Build history of the part. All positions in model axes, mm. A direction names the side the tool comes from. Coordinates: 2 decimals unless noted, no trailing zeros. Loops run counter-clockwise (first coordinate to the right, second up) from the corner with the lowest first, then second, coordinate; pieces in that order, holes last. Notation, with made-up numbers: (-23.75, 56) - (27.25, 56) arc R30 cw to (27.25, 90) - close; hole circle Ø1 at (-5, 38.5). An arc over 180 degrees is marked (long way). One line per item, written item: value.
Autodesk Inventor part; units mm, degrees
ref_plane "YZ Plane" through (0, 0, 0) normal (1, 0, 0) x (0, 1, 0)
ref_plane "XZ Plane" through (0, 0, 0) normal (0, 1, 0) x (-1, 0, 0)
ref_plane "XY Plane" through (0, 0, 0) normal (0, 0, 1) x (1, 0, 0)
sketch "Sketch1" plane through (0, 0, 0) normal (1, 0, 0) x (0, 1, 0)
  line L0 (0, 0) -> (-72, 0)
  line L1 (-80, -8) -> (-80, -72)
  line L2 (-72, -80) -> (0, -80)
  arc A0 (-72, 0) -> (-80, -8) centre (-72, -8) ccw
  arc A1 (-80, -72) -> (-72, -80) centre (-72, -72) ccw
  point P0 (-80, 0)
  point P1 (-80, -80)
  dimension "d0" = 80
  dimension "d1" = 80
  dimension "d2" = 80
  dimension "d3" = 8
sketch "Sketch2" plane through (0, 0, 0) normal (0, 1, 0) x (-1, 0, 0)
  line L0 (-5, 4) -> (5, 4)
  line L1 (5, 4) -> (5, -4)
  line L2 (5, -4) -> (-5, -4)
  line L3 (-5, -4) -> (-5, 4)
  line L4 (-5, 4) -> (5, -4) construction
  line L5 (5, 4) -> (-5, -4) construction
  line L6 (-6.5, -5.5) -> (6.5, -5.5)
  line L7 (6.5, -5.5) -> (6.5, 5.5)
  line L8 (6.5, 5.5) -> (-6.5, 5.5)
  line L9 (-6.5, 5.5) -> (-6.5, -5.5)
  point P0 (0, 0)
  dimension "d4" = 10
  dimension "d5" = 8
  dimension "d6" = 1.5
sweep "Sweep1" add profiles "Sketch2" path "Sketch1"
properties part number "Part323deabril"
Item 1: Cut at A-A, the plane y = -9.5. Write the cut outline in (x, z), then the cut area to 3 significant figures.
Check result:
outline: (-6.5, -85.5) - (6.5, -85.5) - (6.5, -74.5) - (-6.5, -74.5) - close; (-6.5, -5.5) - (6.5, -5.5) - (6.5, 5.5) - (-6.5, 5.5) - close; hole (-5, -84) - (5, -84) - (5, -76) - (-5, -76) - close; hole (-5, -4) - (5, -4) - (5, 4) - (-5, 4) - close
area: 126 mm^2
Item 2: Cut at C-C, the plane z = -60. Write the cut outline in (x, y), then the cut area to 3 significant figures.
Check result:
outline: (-6.5, -85.5) - (6.5, -85.5) - (6.5, -74.5) - (-6.5, -74.5) - close; hole (-5, -84) - (5, -84) - (5, -76) - (-5, -76) - close
area: 63.0 mm^2
Item 3: Cut at D-D, the plane y = -77.5. Write the cut outline in (x, z), then the cut area to 3 significant figures.
Check result:
outline: (-6.5, -84.33) - (6.5, -84.33) - (6.5, 4.33) - (-6.5, 4.33) - close; hole (-5, -82.67) - (5, -82.67) - (5, 2.67) - (-5, 2.67) - close
area: 299 mm^2
Item 4: Cut at B-B, the plane x = -2.5. Write the cut outline in (y, z), then the cut area to 3 significant figures.
Check result:
outline: (-85.5, -72) arc R13.5 ccw to (-72, -85.5) - (0, -85.5) - (0, -84) - (-72, -84) arc R12 cw to (-84, -72) - (-84, -8) arc R12 cw to (-72, 4) - (0, 4) - (0, 5.5) - (-72, 5.5) arc R13.5 ccw to (-85.5, -8) - close; (-76, -72) arc R4 ccw to (-72, -76) - (0, -76) - (0, -74.5) - (-72, -74.5) arc R2.5 cw to (-74.5, -72) - (-74.5, -8) arc R2.5 cw to (-72, -5.5) - (0, -5.5) - (0, -4) - (-72, -4) arc R4 ccw to (-76, -8) - close
area: 699 mm^2
Item 5: Tool access for faces 4 (the face through (-0.091, -73.787, -6.252)), 5 (the face through (0, -37, -4)), 6 (the face through (0.09, -81.65, -81.44)), 7 (the face through (0.07, -74.859, -74.797)): list every direction of +Z, -Z, +X, -X, +Y, -Y with a clear straight run to the whole face (end or side of a thin tool).
Check result:
face 4: +X, -X, +Y
face 5: +Y
face 6: -Z, +X, -X, -Y
face 7: none
Item 6: Probe probe 1 along Z at (x, y) = (0, -13); probe 2 along Z at (x, y) = (-5.25, -49.5); probe 3 along Y at (x, z) = (-3.5, -39.5). List the from-to ranges inside material, lowest first. Write a range as from..to.
Check result:
probe 1: z = -85.5..-84, -76..-74.5, -5.5..-4, 4..5.5
probe 2: z = -85.5..-74.5, -5.5..5.5
probe 3: y = -85.5..-84, -76..-74.5
Item 7: Drop a flat-ended pin along its axis: P1, Ø1, axis at x = 0.5, z = -41, coming from the +Y side. Give the stop position or say it passes through.
Check result:
P1: stops at y = -74.5
Item 8: Pull direction Y, two halves, no side cores. Call faces 1 (the face through (0, -35, -84)), 2 (the face through (0.09, -81.44, 1.65)), 3 (the face through (-0.07, -80.58, 0.39)): released by +Y, released by -Y, zero draft, split by the parting line, or undercut.
Check result:
face 1: zero draft
face 2: released by -Y
face 3: undercut
